Autodesk Inventor part; units mm, degrees
ref_plane "YZ Plane" through (0, 0, 0) normal (1, 0, 0) x (0, 1, 0)
ref_plane "XZ Plane" through (0, 0, 0) normal (0, 1, 0) x (-1, 0, 0)
ref_plane "XY Plane" through (0, 0, 0) normal (0, 0, 1) x (1, 0, 0)
sketch "Sketch1" plane through (0, 0, 0) normal (0, 0, 1) x (1, 0, 0)
  line L0 (0, 0) -> (390, 0)
  line L1 (390, 0) -> (390, 740)
  line L2 (390, 740) -> (0, 740)
  line L3 (0, 740) -> (0, 0)
  dimension "d0" = 390
  dimension "d1" = 740
extrude "Extrusion1" add sketch "Sketch1" along normal blind 20
sketch "Sketch2" plane through (0, 0, 20) normal (0, 0, 1) x (1, 0, 0)
  line L0 (20, 20) -> (370, 20)
  line L1 (370, 20) -> (370, 720)
  line L2 (370, 720) -> (20, 720)
  line L3 (20, 720) -> (20, 20)
  point P0 (0, 0)
  dimension "d6" = 350
  dimension "d7" = 700
extrude "Extrusion2" cut sketch "Sketch2" against normal blind 10
fillet "Fillet1" radius 10 4 edges at (390, 740, 10) (390, 0, 10) (0, 740, 10) (0, 0, 10)
properties part number "Tavla 35x70"
Part model, mm, in its own coordinate system. Give positions to 0.01 mm unless a question says otherwise; leave off trailing zeros. Loops run counter-clockwise (first coordinate to the right, second up) from the corner with the lowest first, then second, coordinate; pieces in that order, holes last.
(1) Band-saw the part on B-B (z = 14.25). Write the cut outline in (x, y), and give its area (3 significant figures).
Return value:
outline: (0, 10) arc R10 ccw to (10, 0) - (380, 0) arc R10 ccw to (390, 10) - (390, 730) arc R10 ccw to (380, 740) - (10, 740) arc R10 ccw to (0, 730) - close; hole (20, 20) - (370, 20) - (370, 720) - (20, 720) - close
area: 43,500 mm2
(2) Band-saw the part on A-A (y = 448). Write the cut outline in (x, z).
Return value:
outline: (0, 0) - (390, 0) - (390, 20) - (370, 20) - (370, 10) - (20, 10) - (20, 20) - (0, 20) - close
(3) Pin check, flat tips, straight feed: pin 1 (10 mm diameter, centred on x = 134, z = 5, fed in from -Y); pin 2 (10 mm diameter, centred on x = 280.5, y = 169.5, fed in from +Z). Stop position of each tip, or through.
Return value:
pin 1: stops at y = 0
pin 2: stops at z = 10
(4) Pull direction Y, two halves, no side cores. Call faces 1 (the flat face through (198, 740, 10)), 2 (the flat face through (390, 365, 10)), 3 (the flat face through (193, 375, 10)): pulls with the +Y half, pulls with the -Y half, needs draft (parallel to the pull), parting line crosses it, or undercut.
Return value:
face 1: pulls with the +Y half
face 2: needs draft
face 3: undercut
(5) Drill centre lines: line 1 along X through (y, z) = (557.5, 12.25); line 2 along Y through (x, z) = (190, 15.75); line 3 along Z through (x, y) = (215, 396). Where is each one in solid material? Low to high.
Return value:
line 1: x = 0 to 20, 370 to 390
line 2: y = 0 to 20, 720 to 740
line 3: z = 0 to 10
(6) Band-saw the part on C-C (x = 77). Write the cut outline in (y, z).
Return value:
outline: (0, 0) - (740, 0) - (740, 20) - (720, 20) - (720, 10) - (20, 10) - (20, 20) - (0, 20) - close
